Geometry: final body of the model. Coordinates: model frame, mm. A direction names the side the tool comes from. Give positions to 0.01 mm unless a question says otherwise; leave off trailing zeros. Write each loop counter-clockwise with the first axis right and the second up, starting at its lowest first coordinate (ties: lowest second). Pieces come first, ordered by that corner, then holes. Notation, with made-up numbers: M 74.5,75.25 L 117.5,75.25 A28 ccw 117.5,95.25 Z; hole C 21,-15 d1. An arc over 180 degrees is marked long. Use a Markdown table: item, result. Add a question column.
1) Section A-A on x = 4.5. Return the cut outline in (y, z), then the cut area to 3 significant figures.
2) Draft query along X for faces 4 (the flat face through (1, 0.7, 1)), 5 (the cylindrical face through (-6.5, 0.7, 0.1)), 6 (the flat face through (1.4, 0, 2.3)). Return one class per face: +X half, -X half, draft (parallel to the pull), parting line (faces both ways), or undercut.
3) Set-up query: faces 1 (the cylindrical face through (-2.44, 2.61, -0.54)), 2 (the cylindrical face through (3.5, 0.8, 0)), 3 (the cylindrical face through (-2.44, 0.35, -0.54)). Return all of +Z, -Z, +X, -X, +Y, -Y with unobstructed straight access to the full face (end or side cutting, diameter ignored); none if empty.
4) Line query: line 1 (Z direction, x = -4.5, y = 0.7); line 2 (Z direction, x = 0, y = 1.05); line 3 (Y direction, x = 5, z = 2). Output: solid intervals per line, ascending.
5) Section C-C on z = 0. State how many separate pieces and enclosed holes the cut face has, then the cut area to 3 significant figures.
6) Section D-D on x = 0. Return the cut outline in (y, z).
7) Pin query (flat end, axial travel): pin 1 (2.5 mm diameter, centred on x = -4.5, z = 0, fed in from +Y); pin 2 (1.5 mm diameter, centred on x = 0.5, z = -1, fed in from -Y); pin 3 (1 mm diameter, centred on y = 2.5, z = 0.5, fed in from +X). Return the tip coordinate at first contact, or that it passes through.
8) Section B-B on y = 0.5. Return the cut outline in (x, z), then the cut area to 3 significant figures.
```python
from build123d import *

# Parameters (mm, degrees)
BASE_SKETCH_W              = 10.95445115
BASE_SKETCH_H              = 7
BASE_EXTRUDE_DEPTH         = 1.5
PROTRUSION_START           = 1.5
F_5MM_DIAMETER_SKETCH_R    = 2.5
PROTRUSION_EXTRUDE_DEPTH   = 2.5
F_5MM_DIAMETER_SKETCH_2_R  = 2.5
F_5MM_BOTTOM_CUT_DEPTH     = 0.7
F_2_0_2_DIAMETER_HOLE1_D   = 2
F_2_5_2_5_DIAMETER_HOLE1_D = 2.5
CUT_EXTRUDE2_START         = 4
F_3MM_DIAMETER_SKETCH_R    = 1.5
CUT_EXTRUDE2_DEPTH         = 2.5


with BuildPart() as part:
    # Base Sketch → Base Extrude (new body)
    with BuildSketch(Plane(origin=(0, 0, 0), x_dir=(1, 0, 0), z_dir=(0, 1, 0))):
        Rectangle(BASE_SKETCH_W, BASE_SKETCH_H)
        with BuildLine():
            ThreePointArc((-5.477225575, -3.5), (-6.5, 0), (-5.477225575, 3.5))
            Line((-5.477225575, 3.5), (-5.477225575, -3.5))
        make_face()
        with BuildLine():
            ThreePointArc((5.477225575, 3.5), (6.5, 0), (5.477225575, -3.5))
            Line((5.477225575, -3.5), (5.477225575, 3.5))
        make_face()
    extrude(amount=BASE_EXTRUDE_DEPTH)

    # 5mm diameter Sketch → Protrusion Extrude (add)
    with BuildSketch(Plane(origin=(0, 0, 0), x_dir=(1, 0, 0), z_dir=(0, 1, 0)).offset(PROTRUSION_START)):
        with Locations(Location((0, 0, 0), (0, 0, 270))):
            Circle(F_5MM_DIAMETER_SKETCH_R)
    extrude(amount=PROTRUSION_EXTRUDE_DEPTH)

    # 5mm diameter Sketch<2> → 5mm Bottom Cut (cut)
    with BuildSketch(Plane(origin=(0, 0, 0), x_dir=(1, 0, 0), z_dir=(0, 1, 0))):
        with Locations(Location((0, 0, 0), (0, 0, 270))):
            Circle(F_5MM_DIAMETER_SKETCH_2_R)
    extrude(amount=F_5MM_BOTTOM_CUT_DEPTH, mode=Mode.SUBTRACT)

    # Chamfer1: read off the stored shape, not the designer's step
    # Chamfer1 outline → Chamfer1 (revolve, cut)
    with BuildSketch(Plane.XY):
        Polygon((2.5, 4), (2.25, 4), (2.5, 3.75), align=None)
    revolve(axis=Axis((0, 0, 0), (0, 1, 0)), mode=Mode.SUBTRACT)

    # Ø2.0 (2) Diameter Hole1 (through all)
    with Locations(Plane(origin=(0, 0, 0), x_dir=(-1, 0, 0), z_dir=(0, -1, 0))):
        with Locations((4.5, 0), (-4.5, 0)):
            Hole(F_2_0_2_DIAMETER_HOLE1_D / 2)

    # Ø2.5 (2.5) Diameter Hole1 (through all)
    with Locations(Plane(origin=(0, 0.7, 0), x_dir=(-1, 0, 0), z_dir=(0, -1, 0))):
        with Locations((0, 0)):
            Hole(F_2_5_2_5_DIAMETER_HOLE1_D / 2)

    # 3mm Diameter Sketch → Cut-Extrude2 (cut)
    with BuildSketch(Plane(origin=(0, 0, 0), x_dir=(1, 0, 0), z_dir=(0, 1, 0)).offset(CUT_EXTRUDE2_START)):
        with Locations(Location((0, 0, 0), (0, 0, 270))):
            Circle(F_3MM_DIAMETER_SKETCH_R)
    extrude(amount=-CUT_EXTRUDE2_DEPTH, mode=Mode.SUBTRACT)


solid = part.part
```
Found:
| question | item | result |
|---|---|---|
| 1 | outline | M 0,-3.5 L 1.5,-3.5 L 1.5,-1 L 0,-1 Z; M 0,1 L 1.5,1 L 1.5,3.5 L 0,3.5 Z |
| 1 | area | 7.50 mm² |
| 2 | face 4 | undercut |
| 2 | face 5 | -X half |
| 2 | face 6 | draft |
| 3 | face 1 | +Y |
| 3 | face 2 | +Y, -Y |
| 3 | face 3 | -Y |
| 4 | line 1 | -3.5 to -1, 1 to 3.5 |
| 4 | line 2 | -3.5 to -1.25, 1.25 to 3.5 |
| 4 | line 3 | 0 to 1.5 |
| 5 | separate pieces | 4 |
| 5 | enclosed holes | 0 |
| 5 | area | 12.9 mm² |
| 6 | outline | M 0,-3.5 L 1.5,-3.5 L 1.5,-2.5 L 3.75,-2.5 L 4,-2.25 L 4,-1.5 L 1.5,-1.5 L 1.5,-1.25 L 0.7,-1.25 L 0.7,-2.5 L 0,-2.5 Z; M 0,2.5 L 0.7,2.5 L 0.7,1.25 L 1.5,1.25 L 1.5,1.5 L 4,1.5 L 4,2.25 L 3.75,2.5 L 1.5,2.5 L 1.5,3.5 L 0,3.5 Z |
| 7 | pin 1 | y = 1.5 |
| 7 | pin 2 | y = 0.7 |
| 7 | pin 3 | x = 2.5 |
| 8 | outline | M -5.48,-3.5 L 5.48,-3.5 A6.5 ccw 5.48,3.5 L -5.48,3.5 A6.5 ccw Z; hole C -4.5,0 d2; hole C 0,0 d5; hole C 4.5,0 d2 |
| 8 | area | 60.5 mm² |
